Here's how the part is built. I have some questions about the finished solid (model axes, mm). Round coordinates to 2 decimals unless told otherwise and drop trailing zeros. Order: outer loops, then holes, each group sorted by start corner. A loop starts at its lowest first (then second) coordinate and runs counter-clockwise, first axis right, second up. Notation, with made-up numbers: (-39, 79) -> (-19, 79) arc R15 cw to (-19, 95) -> close; hole circle Ø5 at (51.5, 29). An arc over 180 degrees is marked (long way). One line per item, written item: value.
```python
from build123d import *

# Parameters (mm, degrees)
SKETCH_1_W          = 106
SKETCH_1_H          = 16
EXTRUDE_1_DEPTH     = 1.5
SKETCH_2_R          = 2
CUT_EXTRUDE_1_DEPTH = 55.536684901


with BuildPart() as part:
    # 스케치1 → 보스-돌출1 (new, symmetric)
    with BuildSketch(Plane(origin=(0, 0, 0), x_dir=(1, 0, 0), z_dir=(0, 1, 0))):
        Rectangle(SKETCH_1_W, SKETCH_1_H)
    extrude(amount=EXTRUDE_1_DEPTH, both=True)

    # 스케치2 → 컷-돌출1 (cut, through all)
    with BuildSketch(Plane(origin=(0, 1.5, 4.5), x_dir=(-1, 0, 0), z_dir=(0, -1, 0))):
        with Locations(Location((0, 4.5, 0), (0, 0, 90))):
            Circle(SKETCH_2_R)
        with Locations(Location((50, 4.5, 0), (0, 0, 90))):
            Circle(SKETCH_2_R)
        with Locations(Location((-50, 4.5, 0), (0, 0, 90))):
            Circle(SKETCH_2_R)
    extrude(amount=CUT_EXTRUDE_1_DEPTH, mode=Mode.SUBTRACT)


solid = part.part
```
Q1. I want a section at B-B on z = 0. Write out the boundary of the cut face in (x, y).
Answers:
outline: (-53, -1.5) -> (-52, -1.5) -> (-52, 1.5) -> (-53, 1.5) -> close; (-48, -1.5) -> (-2, -1.5) -> (-2, 1.5) -> (-48, 1.5) -> close; (2, -1.5) -> (48, -1.5) -> (48, 1.5) -> (2, 1.5) -> close; (52, -1.5) -> (53, -1.5) -> (53, 1.5) -> (52, 1.5) -> close
Q2. I want a section at A-A on x = 50. Write out the boundary of the cut face in (y, z).
Answers:
outline: (-1.5, -8) -> (1.5, -8) -> (1.5, -2) -> (-1.5, -2) -> close; (-1.5, 2) -> (1.5, 2) -> (1.5, 8) -> (-1.5, 8) -> close
Q3. If we mould it in two halves opening along Z, with no side actions, what happens to faces 1 (the face through (53, 0, 0)), 2 (the face through (-51.774, 0.021, -0.923)), 3 (the face through (-1, 0, 8))? For each: pulls with the +Z half, pulls with the -Z half, needs draft (parallel to the pull), parting line crosses it, or undercut.
Answers:
face 1: needs draft
face 2: undercut
face 3: pulls with the +Z half
Q4. I want a section at C-C on y = -1. Write out the boundary of the cut face in (x, z).
Answers:
outline: (-53, -8) -> (53, -8) -> (53, 8) -> (-53, 8) -> close; hole circle Ø4 at (-50, 0); hole circle Ø4 at (0, 0); hole circle Ø4 at (50, 0)
Q5. I need wall thicknesses on line 1 along X through (y, z) = (-0.55, 0); line 2 along X through (y, z) = (0.1, 1.75); line 3 along Z through (x, y) = (50, -0.1). Which ranges of each line are inside material? Lowest first, please.
Answers:
line 1: -53 to -52, -48 to -2, 2 to 48, 52 to 53
line 2: -53 to -50.97, -49.03 to -0.97, 0.97 to 49.03, 50.97 to 53
line 3: -8 to -2, 2 to 8
